Drawing for the job (mm, zero at the part's lowest x, y, z). A direction names the side the tool comes from. Coordinates: 2 decimals unless noted, no trailing zeros. Loops run counter-clockwise (first coordinate to the right, second up) from the corner with the lowest first, then second, coordinate; pieces in that order, holes last. Notation, with made-up numbers: (-34.75, 64.25) -> (23.25, 64.25) arc R9 cw to (23.25, 81.25) -> close; hole circle Ø11 at (67.5, 43). An arc over 180 degrees is marked (long way). Write each question's results on one line, items separated by ' | '.
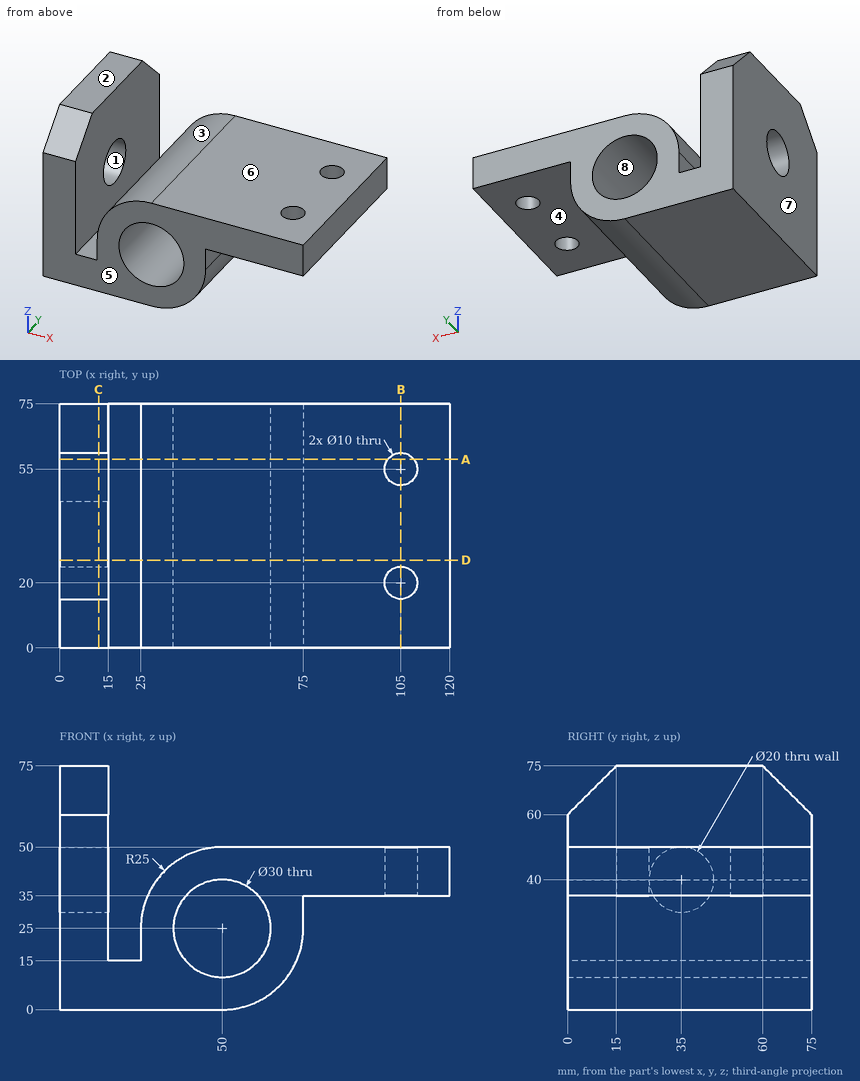
1) Slice it at C-C (x = 12). Write the cut outline in (y, z).
Outcome:
outline: (0, 0) -> (75, 0) -> (75, 60) -> (60, 75) -> (15, 75) -> (0, 60) -> close; hole circle Ø20 at (35, 40)
2) Slice it at A-A (y = 58). Write the cut outline in (x, z), then the cut area to 3 significant figures.
Outcome:
outline: (0, 0) -> (50, 0) arc R25 ccw to (75, 25) -> (75, 35) -> (101, 35) -> (101, 50) -> (50, 50) arc R25 ccw to (25, 25) -> (25, 15) -> (15, 15) -> (15, 75) -> (0, 75) -> close; (109, 35) -> (120, 35) -> (120, 50) -> (109, 50) -> close; hole circle Ø30 at (50, 25) | area: 3,350 mm^2
3) Which spindle directions (+Z, -Z, +X, -X, +Y, -Y) get a long thin tool onto all of the face, cutting with end or side? Do the marked faces 1, 2, 3, 4 and 5. Say none if no direction does.
Outcome:
face 1: -X | face 2: +Z, +X, -X, +Y, -Y | face 3: +Z, +Y, -Y | face 4: -Z, +X, +Y, -Y | face 5: +Z, -Z, +X, -X, -Y
4) Pin check, flat tips, straight feed: pin 1 (9 mm diameter, centred on x = 105, y = 20, fed in from -Z); pin 2 (5 mm diameter, centred on y = 10, z = 25, fed in from +X); pin 3 (13 mm diameter, centred on x = 105, y = 55, fed in from +Z); pin 4 (2 mm diameter, centred on x = 45, y = 65.5, fed in from +Z). Stop position of each tip, or through.
Outcome:
pin 1: passes through | pin 2: stops at x = 75 | pin 3: stops at z = 50 | pin 4: stops at z = 49.68
5) Slice it at B-B (x = 105). Write the cut outline in (y, z).
Outcome:
outline: (0, 35) -> (15, 35) -> (15, 50) -> (0, 50) -> close; (25, 35) -> (50, 35) -> (50, 50) -> (25, 50) -> close; (60, 35) -> (75, 35) -> (75, 50) -> (60, 50) -> close
6) Drill centre lines: L1, parallel to Z at x = 50, y = 28; L2, parallel to Z at x = 11, y = 35; L3, parallel to Y at x = 105, z = 39.75. Where is each one in solid material? Low to high. Write a range as from..to.
Outcome:
L1: z = 0..10, 40..50 | L2: z = 0..30, 50..75 | L3: y = 0..15, 25..50, 60..75
7) Two-plate mould, pull along X, no slides. Class the marked faces 6, 7 and 8: pulls with the +X half, pulls with the -X half, needs draft (parallel to the pull), parting line crosses it, or undercut.
Outcome:
face 6: needs draft | face 7: pulls with the -X half | face 8: undercut
8) Slice it at D-D (y = 27). Write the cut outline in (x, z).
Outcome:
outline: (0, 0) -> (50, 0) arc R25 ccw to (75, 25) -> (75, 35) -> (120, 35) -> (120, 50) -> (50, 50) arc R25 ccw to (25, 25) -> (25, 15) -> (15, 15) -> (15, 34) -> (0, 34) -> close; (0, 46) -> (15, 46) -> (15, 75) -> (0, 75) -> close; hole circle Ø30 at (50, 25)
